Read the model definition and answer for the solid it produces. Units are mm, in the model's axes. A direction names the side the tool comes from. Coordinates: 2 decimals unless noted, no trailing zeros. Loops run counter-clockwise (first coordinate to the right, second up) from the corner with the lowest first, then second, coordinate; pieces in that order, holes last. Notation, with made-up numbers: (56, 72.25) - (94, 72.25) arc R13 cw to (94, 86.25) - close; hole circle Ø2 at (-35, 26.25). An arc over 180 degrees is marked (long way). One line per item, written item: value. Start each with the question number.
from build123d import *

# Parameters (mm, degrees)
EXTRUDE_1_DEPTH      = 42
SHELL_1_T            = -1.5
EXTRUDE_4_DEPTH      = 25
FILLET_2_R           = 3
CUT_EXTRUDE_3_DEPTH  = 126.73384588089242
CUT_EXTRUDE_4_DEPTH  = 126.73384588089242
EXTRUDE_5_DEPTH      = 4
CUT_EXTRUDE_7_DEPTH  = 3
CUT_EXTRUDE_START    = -0.1
CUT_EXTRUDE_12_DEPTH = 0.1
SKETCH_18_R          = 3.0000000000000018
SKETCH_18_R_2        = 2.0000000000000036
EXTRUDE_6_DEPTH      = 5
FILLET_3_R           = 3
SKETCH_22_W          = 3
SKETCH_22_H          = 3.000000000000014
CUT_EXTRUDE_13_DEPTH = 3
SKETCH_23_W          = 3.000000000000007
SKETCH_23_H          = 3.000000000000014
CUT_EXTRUDE_14_DEPTH = 3
FILLET_4_R           = 3


with BuildPart() as part:
    # 草图1 → 凸台-拉伸1 (new body)
    with BuildSketch(Plane(origin=(0, 0, 0), x_dir=(1, 0, 0), z_dir=(0, 1, 0))):
        Polygon((-53.000000000000014, 53), (52.999999999999986, 53), (53, -53), (-53, -53), align=None)
    extrude(amount=EXTRUDE_1_DEPTH)

    # 抽壳1
    shell_1_openings = [part.faces().sort_by_distance(p)[0] for p in [
        (0, 42, 0),
    ]]
    offset(amount=SHELL_1_T, openings=shell_1_openings, kind=Kind.INTERSECTION)

    # 草图3 → 凸台-拉伸4 (add)
    with BuildSketch(Plane(origin=(0, 1.5, 0), x_dir=(1, 0, 0), z_dir=(0, 1, 0))):
        Polygon((-6.500000000000012, 41.49999999999999), (-6.500000000000003, -41.49999999999999), (-5.500000000000003, -41.49999999999999), (-5.5000000000000036, 41.49999999999999), align=None)
        Polygon((1.4999999999999944, 41.49999999999999), (1.5000000000000053, -41.49999999999999), (0.5000000000000043, -41.49999999999999), (0.4999999999999944, 41.49999999999999), align=None)
    extrude(amount=EXTRUDE_4_DEPTH)

    # 圆角2
    fillet_2_edges = [part.edges().sort_by_distance(p)[0] for p in [
        (51.5, 21.75, 51.5),
        (51.499999999999986, 21.75, -51.5),
        (-51.500000000000014, 21.75, -51.5),
        (-51.5, 21.75, 51.5),
        (0, 0, 53),
        (-53.00000000000001, 0, 0),
        (-1.421e-14, 0, -53),
        (52.99999999999999, 0, 0),
        (53, 21, 53),
        (-53, 21, 53),
        (-53.000000000000014, 21, -53),
        (52.999999999999986, 21, -53),
    ]]
    fillet(fillet_2_edges, radius=FILLET_2_R)

    # 草图6 → 切除-拉伸3 (cut, through all)
    with BuildSketch(Plane.XY.offset(53)):
        Polygon((-53, 36.00000000000001), (2.0000000000000018, 36.00000000000001), (31.393876913398135, 42), (-53, 42), align=None)
    extrude(amount=-CUT_EXTRUDE_3_DEPTH, mode=Mode.SUBTRACT)

    # 草图7 → 切除-拉伸4 (cut, through all)
    with BuildSketch(Plane.XY.offset(53)):
        with BuildLine():
            Line((13.866100098640908, 33.319053909073325), (36.958961236370065, 38.032864449771985))
            ThreePointArc((36.958961236370065, 38.032864449771985), (31.499999999999993, 5.853571800517756), (13.866100098640908, 33.319053909073325))
        make_face()
    extrude(amount=-CUT_EXTRUDE_4_DEPTH, mode=Mode.SUBTRACT)

    # 草图8 → 凸台-拉伸5 (add)
    with BuildSketch(Plane(origin=(0, 0, 51.5), x_dir=(-1, 0, 0), z_dir=(0, 0, -1))):
        Polygon((-45.32050807568879, 13.00000000000003), (-44.021469970012134, 13.750000000000028), (-11.978530029987853, 13.750000000000032), (-10.679491924311197, 13.000000000000034), (-10.679491924311197, 1.5000000000000053), (-45.32050807568879, 1.5000000000000009), align=None)
    extrude_5 = extrude(amount=EXTRUDE_5_DEPTH)

    # 草图10 → 切除-拉伸7 (cut)
    with BuildSketch(Plane(origin=(0, 0, 51.5), x_dir=(-1, 0, 0), z_dir=(0, 0, -1))):
        with BuildLine():
            Line((-45.3205080756888, 13.000000000000043), (-27.999999999999996, 23))
            Line((-27.999999999999996, 23), (-10.679491924311197, 13.000000000000043))
            ThreePointArc((-10.679491924311197, 13.000000000000043), (-28, 2.9999999999999964), (-45.3205080756888, 13.000000000000043))
        make_face()
    cut_extrude_7 = extrude(amount=CUT_EXTRUDE_7_DEPTH, mode=Mode.SUBTRACT)

    # 镜向1: 凸台-拉伸5, 切除-拉伸7 across plane
    add(extrude_5.mirror(Plane.XY))
    add(cut_extrude_7.mirror(Plane.XY), mode=Mode.SUBTRACT)

    # 草图17 → 切除-拉伸12 (cut)
    with BuildSketch(Plane(origin=(0, 1.5, 0), x_dir=(1, 0, 0), z_dir=(0, 1, 0)).offset(CUT_EXTRUDE_START)):
        with BuildLine():
            Line((10.679491924311197, 47.5), (10.679491924311197, 51.5))
            Line((10.679491924311197, 51.5), (-48.50000000000001, 51.5))
            ThreePointArc((-48.50000000000001, 51.5), (-50.62132034355965, 50.62132034355964), (-51.500000000000014, 48.49999999999999))
            Line((-51.500000000000014, 48.49999999999999), (-51.5, -48.49999999999999))
            ThreePointArc((-51.5, -48.49999999999999), (-50.62132034355964, -50.62132034355964), (-48.49999999999999, -51.5))
            Line((-48.49999999999999, -51.5), (10.679491924311197, -51.5))
            Line((10.679491924311197, -51.5), (10.679491924311197, -47.5))
            Line((10.679491924311197, -47.5), (45.32050807568879, -47.5))
            Line((45.32050807568879, -47.5), (45.32050807568879, -51.5))
            Line((45.32050807568879, -51.5), (48.49999999999999, -51.5))
            ThreePointArc((48.49999999999999, -51.5), (50.62132034355964, -50.62132034355964), (51.5, -48.49999999999999))
            Line((51.5, -48.49999999999999), (51.499999999999986, 48.49999999999999))
            ThreePointArc((51.499999999999986, 48.49999999999999), (50.621320343559624, 50.62132034355964), (48.49999999999998, 51.5))
            Line((48.49999999999998, 51.5), (45.32050807568879, 51.5))
            Line((45.32050807568879, 51.5), (45.32050807568879, 47.5))
            Line((45.32050807568879, 47.5), (10.679491924311197, 47.5))
        make_face()
        Polygon((1.4999999999999944, 41.49999999999999), (0.4999999999999944, 41.49999999999999), (0.5000000000000043, -41.49999999999999), (1.5000000000000053, -41.49999999999999), align=None, mode=Mode.SUBTRACT)
        Polygon((-5.5000000000000036, 41.49999999999999), (-6.500000000000012, 41.49999999999999), (-6.500000000000003, -41.49999999999999), (-5.500000000000003, -41.49999999999999), align=None, mode=Mode.SUBTRACT)
    extrude(amount=CUT_EXTRUDE_12_DEPTH, mode=Mode.SUBTRACT)

    # 草图18 → 凸台-拉伸6 (add)
    # profile 1 of 2: a face of its own
    with BuildSketch(Plane(origin=(0, 1.4, 0), x_dir=(1, 0, 0), z_dir=(0, 1, 0))):
        with Locations((-48.50000000000001, 48.49999999999999)):
            Circle(SKETCH_18_R)
        with Locations(Location((-48.50000000000001, 48.49999999999999, 0), (0, 0, 270))):
            Circle(SKETCH_18_R_2, mode=Mode.SUBTRACT)
    # profile 2 of 2: a face of its own
    with BuildSketch(Plane(origin=(0, 1.4, 0), x_dir=(1, 0, 0), z_dir=(0, 1, 0))):
        with Locations((48.49999999999998, 48.49999999999999)):
            Circle(SKETCH_18_R)
        with Locations(Location((48.49999999999998, 48.49999999999999, 0), (0, 0, 270))):
            Circle(SKETCH_18_R_2, mode=Mode.SUBTRACT)
    extrude_6 = extrude(amount=EXTRUDE_6_DEPTH)

    # 镜向2: 凸台-拉伸6 across plane
    add(extrude_6.mirror(Plane.XY))

    # 圆角3
    fillet_3_edges = [part.edges().sort_by_distance(p)[0] for p in [
        (46.91025403784438, 1.4, -51.5),
        (51.49999999999999, 1.4, 0),
        (46.910254037844396, 1.4, 51.5),
        (-18.910254037844396, 1.4, 51.5),
        (-51.50000000000001, 1.4, 0),
        (-18.910254037844407, 1.4, -51.5),
    ]]
    fillet(fillet_3_edges, radius=FILLET_3_R)

    # 草图22 → 切除-拉伸13 (cut)
    with BuildSketch(Plane(origin=(1.49e-15, 13.750000000000034, 0), x_dir=(1, -1.1e-16, 0), z_dir=(1.1e-16, 1, 0))):
        with Locations((12.179491924311202, 50)):
            Rectangle(SKETCH_22_W, SKETCH_22_H)
    cut_extrude_13 = extrude(amount=-CUT_EXTRUDE_13_DEPTH, mode=Mode.SUBTRACT)

    # 草图23 → 切除-拉伸14 (cut)
    with BuildSketch(Plane(origin=(1.49e-15, 13.750000000000034, 0), x_dir=(1, -1.1e-16, 0), z_dir=(1.1e-16, 1, 0))):
        with Locations((43.82050807568879, 50)):
            Rectangle(SKETCH_23_W, SKETCH_23_H)
    cut_extrude_14 = extrude(amount=-CUT_EXTRUDE_14_DEPTH, mode=Mode.SUBTRACT)

    # 镜向3: 切除-拉伸13, 切除-拉伸14 across plane
    add(cut_extrude_13.mirror(Plane.XY), mode=Mode.SUBTRACT)
    add(cut_extrude_14.mirror(Plane.XY), mode=Mode.SUBTRACT)

    # 圆角4
    fillet_4_edges = [part.edges().sort_by_distance(p)[0] for p in [
        (-5.5000000000000036, 1.4, 0),
        (-6.500000000000008, 1.4, 0),
        (1.5, 1.4, 0),
        (0.49999999999999933, 1.4, 0),
    ]]
    fillet(fillet_4_edges, radius=FILLET_4_R - 0.0001)  # a hair under: the kernel refuses the full size


solid = part.part
1) Flat-ended cylindrical pins translate along their axes: P1, Ø5, axis at x = -48.5, z = 48.5, coming from the +Y side; P2, Ø5, axis at x = -19.5, z = 8, coming from the +Y side; P3, Ø0.8, axis at x = 31, z = -48, coming from the +Y side. Find the tip coordinate at first contact, or state that the pin passes through.
2) Section B-B, the plane x = -35.5 is taken. Determine the outline of the cut face in (y, z).
3) Section A-A, the plane y = 23 is taken. State how many separate pieces and enclosed holes the cut face has, and give its area (3 significant figures).
4) For faces 4 (the flat face through (-6, 12, -41.5)), 5 (the cylindrical face through (32.07, 5.98, -52.24)), 6 (the flat face through (16.491, 38.958, 52.26)), determine the directions among +Z, -Z, +X, -X, +Y, -Y from which every point of the face is accessible in a straight line to the end or side of a thin tool.
5) Section D-D, the plane x = 28 is taken. Determine the outline of the cut face in (y, z), and give its area (3 significant figures).
6) Straight lines are drawn through the part: L1, parallel to X at y = 6.5, z = -48; L2, parallel to Z at x = 48.5, y = 3.4; L3, parallel to X at y = 22.5, z = 37.5. For each, find the intervals that lie inside material, in ascending order.
7) Determine the mould class of faces 1 (the cylindrical face through (52.14, 0.9, 0.7)), 2 (the cylindrical face through (46.31, 3.86, -46.45)), 3 (the cylindrical face through (-52.14, 0.9, -0.7)) for opening direction X: released by +X, released by -X, zero draft, split by the parting line, or undercut.
Answer below:
1. P1: y = 6.4
1. P2: y = 1.4
1. P3: y = 13.75
2. outline: (0, -50) arc R3 ccw to (3, -53) - (36, -53) - (36, -51.5) - (4.4, -51.5) arc R3 cw to (1.4, -48.5) - (1.4, 48.5) arc R3 cw to (4.4, 51.5) - (36, 51.5) - (36, 53) - (3, 53) arc R3 ccw to (0, 50) - close
3. separate pieces: 4
3. enclosed holes: 0
3. area: 688 mm2
4. face 4: +Y
4. face 5: -Z
4. face 6: +Z, -Z, -X, +Y
5. outline: (0, -50) arc R3 ccw to (3, -53) - (5.5, -53) - (5.5, -51.5) - (3, -51.5) - (3, -48.5) - (13.75, -48.5) - (13.75, -47.5) - (1.4, -47.5) - (1.4, 47.5) - (13.75, 47.5) - (13.75, 48.5) - (3, 48.5) - (3, 51.5) - (5.5, 51.5) - (5.5, 53) - (3, 53) arc R3 ccw to (0, 50) - close; (36.2, -53) - (41.31, -53) - (41.31, -51.5) - (36.2, -51.5) - close; (36.2, 51.5) - (41.31, 51.5) - (41.31, 53) - (36.2, 53) - close
5. area: 206 mm2
6. L1: -53 to -51.5, 10.68 to 45.32, 51.5 to 53
6. L2: -53 to -50.5, -46.5 to -45.5, 45.5 to 46.5, 50.5 to 53
6. L3: -53 to -51.5, -6.5 to -5.5, 0.5 to 1.5, 51.5 to 53
7. face 1: released by +X
7. face 2: undercut
7. face 3: released by -X
